The model under review builds one solid part; all positions refer to its coordinate system, in mm. A direction names the side the tool comes from. Coordinates: 2 decimals unless noted, no trailing zeros. Loops run counter-clockwise (first coordinate to the right, second up) from the corner with the lowest first, then second, coordinate; pieces in that order, holes last. Notation, with made-up numbers: (22, -25.5) - (45, -25.5) arc R21 ccw to (45, 0.5) - close; hole circle Ø7 at (1.25, 82.25). An arc over 180 degrees is marked (long way). Answer in a Markdown table with one row per item. Add a question column.
(1) Machinability: for faces 3 (the cylindrical face through (-0.867, -3.905, 1.973)), 4 (the flat face through (-4, -3, 0.25)), which of the approach directions +Z, -Z, +X, -X, +Y, -Y give a long, thin tool a straight path to every point of the face, cutting with its end or side? Answer none if there is none.
(2) For line 1 along Y through (x, z) = (0, 3.85); line 2 along X through (y, z) = (2.5, 0.2); line 3 along Y through (x, z) = (0, 2.1), list the stretches that pass through material, from the lowest coordinate up.
(3) For P1, Ø4, axis at x = 2.5, y = -1, coming from the +Z side; P2, Ø2, axis at x = 4, z = 2, coming from the +Y side; P3, Ø1.5, axis at y = -1.5, z = 3.5, coming from the +X side; P4, Ø1, axis at x = 1, z = 3, coming from the +Y side, all flat-tipped, find the tip position at first contact; note any pin that passes through.
(4) We need section C-C on z = 1.9. Write out the cut boundary in (x, y), plus the area to 3 significant figures.
(5) Mouldability with a two-part tool opening along Y and no side actions: class faces 1 (the flat face through (4, -3, 3.75)), 2 (the cylindrical face through (6.466, -2.681, 1.973)) as +Y half, -Y half, draft (parallel to the pull), parting line (faces both ways), or undercut.
from build123d import *

# Parameters (mm, degrees)
SKETCH1_R           = 7
SKETCH1_R_2         = 4
BOSS_EXTRUDE1_DEPTH = 4
SKETCH2_R           = 6.4
SKETCH2_R_2         = 4.6
CUT_EXTRUDE1_DEPTH  = 0.25
SKETCH3_R           = 6.4
SKETCH3_R_2         = 4.6
CUT_EXTRUDE2_DEPTH  = 0.25
FILLET1_R           = 0.1
FILLET2_R           = 0.1


with BuildPart() as part:
    # Sketch1 → Boss-Extrude1 (new body)
    with BuildSketch(Plane.XY):
        Circle(SKETCH1_R)
        Circle(SKETCH1_R_2, mode=Mode.SUBTRACT)
    extrude(amount=BOSS_EXTRUDE1_DEPTH)

    # Sketch2 → Cut-Extrude1 (cut)
    with BuildSketch(Plane.XY.offset(4)):
        Circle(SKETCH2_R)
        Circle(SKETCH2_R_2, mode=Mode.SUBTRACT)
    extrude(amount=-CUT_EXTRUDE1_DEPTH, mode=Mode.SUBTRACT)

    # Sketch3 → Cut-Extrude2 (cut)
    with BuildSketch(Plane(origin=(0, 0, 0), x_dir=(-1, 0, 0), z_dir=(0, 0, -1))):
        Circle(SKETCH3_R)
        Circle(SKETCH3_R_2, mode=Mode.SUBTRACT)
    extrude(amount=-CUT_EXTRUDE2_DEPTH, mode=Mode.SUBTRACT)

    # Fillet1
    fillet1_edges = [part.edges().sort_by_distance(p)[0] for p in [
        (-7, 0, 0),
        (-7, 0, 4),
    ]]
    fillet(fillet1_edges, radius=FILLET1_R)

    # Fillet2
    fillet2_edges = [part.edges().sort_by_distance(p)[0] for p in [
        (-4, 0, 0),
        (-4, 0, 4),
    ]]
    fillet(fillet2_edges, radius=FILLET2_R)


solid = part.part
Outcome:
| question | item | result |
|---|---|---|
| 1 | face 3 | +Z, -Z |
| 1 | face 4 | -Z |
| 2 | line 1 | -7 to -6.4, -4.6 to -4, 4 to 4.6, 6.4 to 7 |
| 2 | line 2 | -6.54 to -5.89, -3.86 to -3.12, 3.12 to 3.86, 5.89 to 6.54 |
| 2 | line 3 | -7 to -4, 4 to 7 |
| 3 | P1 | z = 4 |
| 3 | P2 | y = 6.32 |
| 3 | P3 | x = 6.96 |
| 3 | P4 | y = 6.98 |
| 4 | outline | circle Ø14 at (0, 0); hole circle Ø8 at (0, 0) |
| 4 | area | 104 mm² |
| 5 | face 1 | undercut |
| 5 | face 2 | parting line |
